Input: part model. Units: mm. Frame: model coordinates. Coordinates: 2 decimals unless noted, no trailing zeros. Write each loop counter-clockwise with the first axis right and the second up, starting at its lowest first coordinate (ties: lowest second). Pieces come first, ordered by that corner, then holes. Notation, with made-up numbers: (51, -22) - (68, -22) arc R14 ccw to (68, 5) - close; hole circle Ø7 at (-10, 47.5). An arc over 180 degrees is marked (long way). Use CSV: the item, a comma, the result in double quotes.
```python
from build123d import *

# Parameters (mm, degrees)
PLATE_DEPTH                = 3.175
DRIVE_HOLES_D              = 4.064
SKETCH3_R                  = 3.175
TUBE_PIVOT_HOLES_DEPTH     = 521.864531932
BOTTOM_CORNER_CHAMFER_SIZE = 6.35
BOTTOM_CORNER_FILLET_R     = 3.175
CARBON_CAP_HOLES_D         = 4.064


with BuildPart() as part:
    # Sketch2 → Plate (new body)
    with BuildSketch(Plane(origin=(0, 0, 0), x_dir=(0, 0, -1), z_dir=(1, 0, 0))):
        with BuildLine():
            Line((0, 0), (0, 50.8))
            Line((0, 50.8), (38.311002826, 346.167173299))
            ThreePointArc((38.311002826, 346.167173299), (55.900445741, 367.136476127), (82.313788673, 359.96462293))
            Line((82.313788673, 359.96462293), (112.596875039, 326.577445868))
            ThreePointArc((112.596875039, 326.577445868), (119.137016705, 321.404317358), (127, 318.627951872))
            Line((127, 318.627951872), (207.610663713, 304.414116927))
            ThreePointArc((207.610663713, 304.414116927), (218.737141463, 299.493711333), (226.299177538, 289.963522))
            Line((226.299177538, 289.963522), (322.101644923, 80.472956))
            ThreePointArc((322.101644923, 80.472956), (340.846528773, 58.857200401), (368.3, 50.8))
            Line((368.3, 50.8), (368.3, 0))
            Line((368.3, 0), (0, 0))
        make_face()
    extrude(amount=PLATE_DEPTH)

    # Drive Holes (through all)
    with Locations(Plane(origin=(3.175, 0, 0), x_dir=(0, 0, -1), z_dir=(1, 0, 0))):
        with Locations((184.15, 24.60625), (220.717386247, 25.4), (256.023386247, 25.4), (291.329386247, 25.4), (327.905386247, 25.4), (147.582613753, 25.4), (112.276613753, 25.4), (76.970613753, 25.4), (40.394613753, 25.4)):
            Hole(DRIVE_HOLES_D / 2)

    # Sketch3 → Tube Pivot Holes (cut, through all)
    with BuildSketch(Plane(origin=(3.175, 0, 0), x_dir=(0, 0, -1), z_dir=(1, 0, 0))):
        with Locations((63.5, 342.9)):
            Circle(SKETCH3_R)
    extrude(amount=-TUBE_PIVOT_HOLES_DEPTH, mode=Mode.SUBTRACT)

    # Bottom Corner Chamfer
    bottom_corner_chamfer_edges = [part.edges().sort_by_distance(p)[0] for p in [
        (1.5875, 0, 0),
        (1.5875, 0, -368.3),
    ]]
    chamfer(bottom_corner_chamfer_edges, length=BOTTOM_CORNER_CHAMFER_SIZE)

    # Bottom Corner Fillet
    bottom_corner_fillet_edges = [part.edges().sort_by_distance(p)[0] for p in [
        (1.5875, 0, -6.35),
        (1.5875, 0, -361.95),
        (1.5875, 6.35, 0),
        (1.5875, 50.8, 0),
        (1.5875, 50.8, -368.3),
        (1.5875, 6.35, -368.3),
    ]]
    fillet(bottom_corner_fillet_edges, radius=BOTTOM_CORNER_FILLET_R)

    # Carbon Cap Holes (through all)
    with Locations(Plane(origin=(3.175, 0, 0), x_dir=(0, 0, -1), z_dir=(1, 0, 0))):
        with Locations((5.55625, 45.24375), (5.55625, 8.651474106), (362.74375, 45.24375), (362.74375, 8.651474106)):
            Hole(CARBON_CAP_HOLES_D / 2)


solid = part.part
```
(1) Cut plane B-B on y = 279. Return loops of the section in (x, z) (3 decimals), and give its area (3 significant figures).
Check values:
outline,"(0, -231.313) - (3.175, -231.313) - (3.175, -29.599) - (0, -29.599) - close"
area,"640 mm^2"
(2) Pin query (flat end, axial travel): pin 1 Ø4.5 at (y, z) = (45.24, -5.56) entering from +X (3 decimals); pin 2 Ø1 at (x, z) = (2.5, -145) entering from +Y. Return the tip coordinate at first contact, or that it passes through.
Check values:
pin 1,"x = 3.175"
pin 2,"y = 315.54"
(3) Ray query, probe 1 along Y at (x, z) = (1.3, -63.5) (3 decimals); probe 2 along Y at (x, z) = (0.35, -113); probe 3 along Y at (x, z) = (2.35, -315). Return the intervals inside material, ascending. Write a range as from..to.
Check values:
probe 1,"0..339.725, 346.075..368.3"
probe 2,"0..23.5, 27.3..326.14"
probe 3,"0..96"
(4) Cut plane C-C on y = 120.5. Return loops of the section in (x, z) (3 decimals), and give its area (3 significant figures).
Check values:
outline,"(0, -303.797) - (3.175, -303.797) - (3.175, -9.041) - (0, -9.041) - close"
area,"936 mm^2"
(5) Cut plane A-A on x = 1.7. State how many separate pieces and enclosed holes the cut face has, and give its area (3 significant figures).
Check values:
separate pieces,"1"
enclosed holes,"14"
area,"89,600 mm^2"
